Can you work these out from the drawing? Everything is in mm from the part's minimum corner. A direction names the side the tool comes from. Coordinates: 2 decimals unless noted, no trailing zeros. Order: outer loops, then holes, each group sorted by start corner. A loop starts at its lowest first (then second) coordinate and runs counter-clockwise, first axis right, second up. Notation, with made-up numbers: (5.5, 18.5) -> (20.5, 18.5) arc R34 cw to (20.5, 48.5) -> close; hole circle Ø11 at (0.5, 83.5). An arc over 180 degrees is marked (long way). Put each result on its own line as item: value. Start each with the question number.
Q1. If we section it at B-B (y = 24): Please give me the cut outline in (x, z), and give its area (3 significant figures).
Q2. For the marked faces 1, 2 and 3, which set-ups out of +Z, -Z, +X, -X, +Y, -Y let a thin tool reach every point of the face, with its end or its side?
Q3. Please list where these lines run through material, in increasing order: line 1 along Z through (x, y) = (42, 9.75); line 2 along Y through (x, z) = (42, 22); line 3 along X through (y, z) = (3.25, 11).
Q4. If we section it at C-C (x = 41): Please give me the cut outline in (y, z).
Q5. Will these pins go through, and if not, where does the flat tip stop? pin 1 (1.2 mm diameter, centred on x = 36, y = 3.5, fed in from -Z); pin 2 (5 mm diameter, centred on x = 7, y = 3.5, fed in from -Z); pin 3 (4 mm diameter, centred on x = 9.5, y = 8, fed in from +Z); pin 4 (1 mm diameter, centred on x = 37.5, z = 30, fed in from -Y).
Q6. If we section it at A-A (z = 25): Please give me the cut outline in (x, y).
Q7. If we section it at D-D (y = 18): Please give me the cut outline in (x, z).
Q8. We'd pull the mould along Y, two halves only. Please class the marked faces 4, 5, 6 and 7: +Y half, -Y half, draft (parallel to the pull), parting line (faces both ways), or undercut.
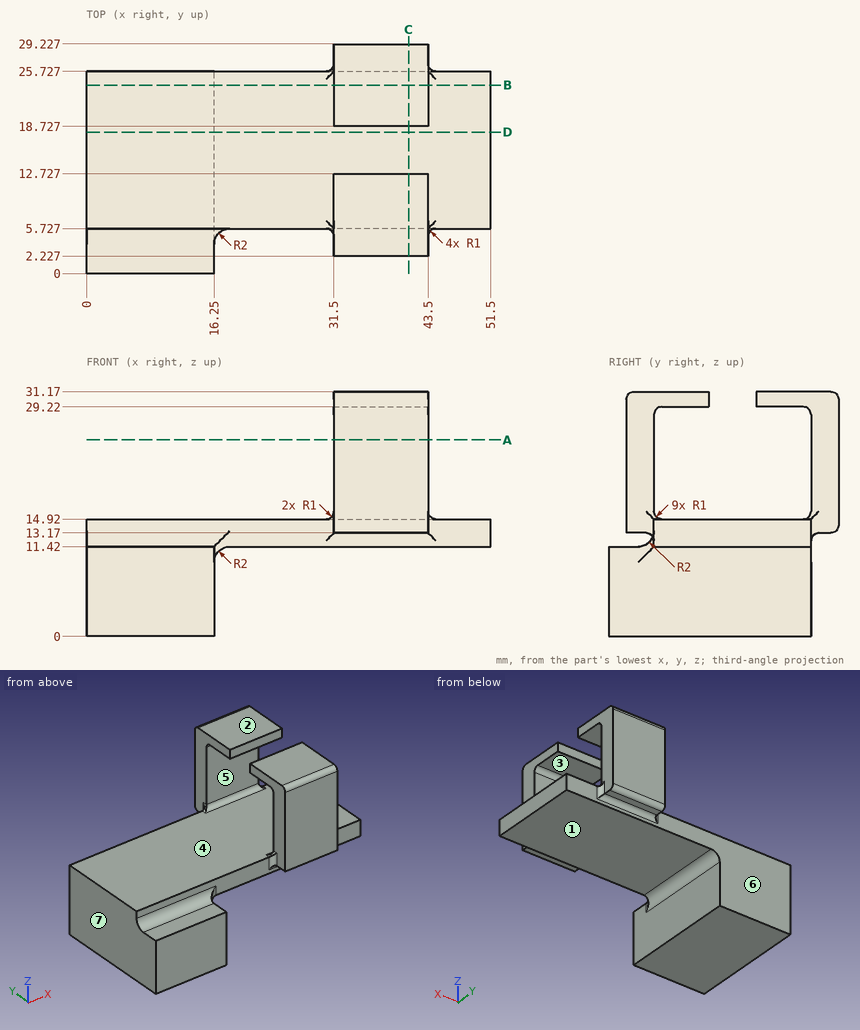
The answers:
1. outline: (0, 0) -> (16.25, 0) -> (16.25, 9.42) arc R2 cw to (18.25, 11.42) -> (51.5, 11.42) -> (51.5, 14.92) -> (0, 14.92) -> close; (31.5, 29.22) -> (43.5, 29.22) -> (43.5, 31.17) -> (31.5, 31.17) -> close
1. area: 390 mm^2
2. face 1: -Z, +X, +Y, -Y
2. face 2: +Z, +X, -X, +Y, -Y
2. face 3: +X, -X
3. line 1: 11.42 to 14.92, 29.22 to 31.17
3. line 2: 2.23 to 5.73, 25.73 to 29.23
3. line 3: 0 to 16.25
4. outline: (2.23, 13.17) -> (4.73, 13.17) arc R1 cw to (5.73, 12.17) -> (5.73, 11.42) -> (25.73, 11.42) -> (25.73, 12.17) arc R1 cw to (26.73, 13.17) -> (28.23, 13.17) arc R1 ccw to (29.23, 14.17) -> (29.23, 30.17) arc R1 ccw to (28.23, 31.17) -> (18.73, 31.17) -> (18.73, 29.22) -> (24.73, 29.22) arc R1 cw to (25.73, 28.22) -> (25.73, 15.92) arc R1 cw to (24.73, 14.92) -> (6.73, 14.92) arc R1 cw to (5.73, 15.92) -> (5.73, 28.22) arc R1 cw to (6.73, 29.22) -> (12.73, 29.22) -> (12.73, 31.17) -> (3.23, 31.17) arc R1 ccw to (2.23, 30.17) -> close
5. pin 1: z = 13.17
5. pin 2: z = 0
5. pin 3: z = 14.92
5. pin 4: y = 2.23
6. outline: (31.5, 2.23) -> (43.5, 2.23) -> (43.5, 5.73) -> (31.5, 5.73) -> close; (31.5, 25.73) -> (43.5, 25.73) -> (43.5, 29.23) -> (31.5, 29.23) -> close
7. outline: (0, 0) -> (16.25, 0) -> (16.25, 9.42) arc R2 cw to (18.25, 11.42) -> (51.5, 11.42) -> (51.5, 14.92) -> (0, 14.92) -> close
8. face 4: undercut
8. face 5: undercut
8. face 6: +Y half
8. face 7: draft
